Part print with two shaded views. Sizes in mm from the minimum x, y, z corner. Give positions to 0.01 mm unless a question says otherwise; leave off trailing zeros. Loops run counter-clockwise (first coordinate to the right, second up) from the corner with the lowest first, then second, coordinate; pieces in that order, holes last. Notation, with made-up numbers: (42, 89) -> (79, 89) arc R19 cw to (79, 107) -> close; hole circle Ø7 at (-34, -35). An arc over 180 degrees is marked (long way). One line per question, with ' | ' between items. Start each with the question number.
(1) Slice it at B-B, the plane z = 1.15. Write the cut outline in (x, y).
(2) Drill centre lines: L1, parallel to Y at x = 28, z = 1.3; L2, parallel to X at y = 8, z = 0.55; L3, parallel to X at y = 12, z = 0.7. Where is each one in solid material? Low to high. Write a range as from..to.
(3) Slice it at A-A, the plane x = 75. Write the cut outline in (y, z).
(4) Slice it at C-C, the plane x = 62. Write the cut outline in (y, z), then the cut area to 3 significant figures.
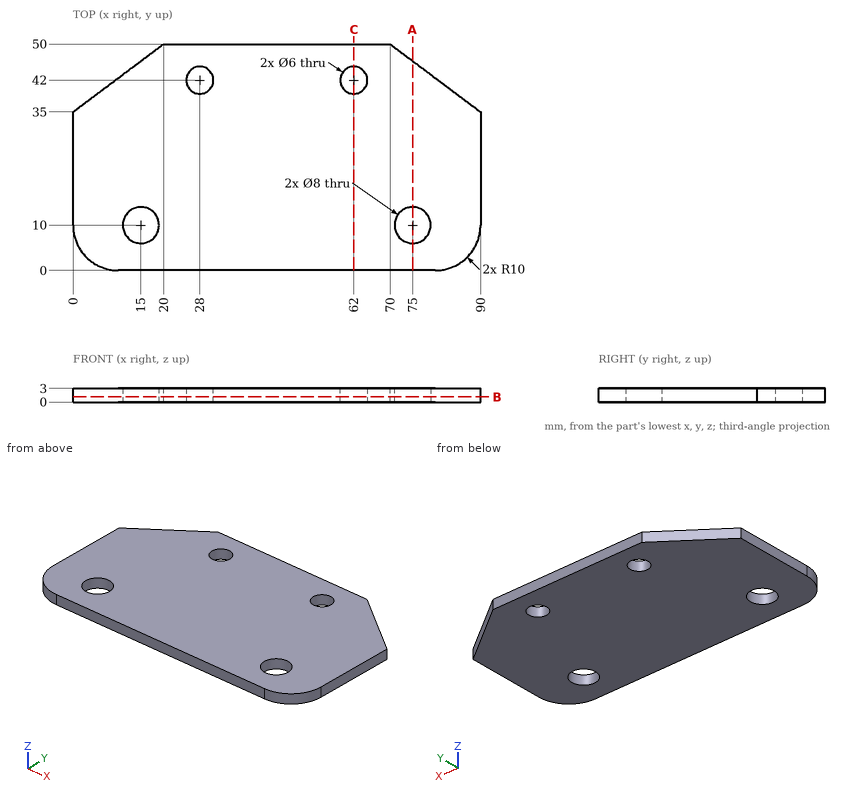
Final values:
1) outline: (0, 10) arc R10 ccw to (10, 0) -> (80, 0) arc R10 ccw to (90, 10) -> (90, 35) -> (70, 50) -> (20, 50) -> (0, 35) -> close; hole circle Ø8 at (15, 10); hole circle Ø6 at (28, 42); hole circle Ø6 at (62, 42); hole circle Ø8 at (75, 10)
2) L1: 0..39, 45..50 | L2: 0.2..11.54, 18.46..71.54, 78.46..89.8 | L3: 0..11.54, 18.46..71.54, 78.46..90
3) outline: (0, 0) -> (6, 0) -> (6, 3) -> (0, 3) -> close; (14, 0) -> (46.25, 0) -> (46.25, 3) -> (14, 3) -> close
4) outline: (0, 0) -> (39, 0) -> (39, 3) -> (0, 3) -> close; (45, 0) -> (50, 0) -> (50, 3) -> (45, 3) -> close | area: 132 mm2
